Part model, mm, in its own coordinate system. A direction names the side the tool comes from. Coordinates: 2 decimals unless noted, no trailing zeros. Order: outer loops, then holes, each group sorted by start corner. A loop starts at its lowest first (then second) coordinate and runs counter-clockwise, first axis right, second up.
from build123d import *

# Parameters (mm, degrees)
SKETCH_1_R               = 19
EXTRUDE_1_DEPTH          = 69
CUT_EXTRUDE_1_DEPTH      = 75.047282192
CUT_EXTRUDE_1_DEPTH_BACK = 75.047282192
SKETCH_4_W               = 20
SKETCH_4_H               = 14
CUT_EXTRUDE_2_DEPTH      = 68.113709479
SKETCH_5_W               = 20
SKETCH_5_H               = 19.031424338
CUT_EXTRUDE_3_DEPTH      = 6
SKETCH_6_R               = 0.75
CUT_EXTRUDE_4_DEPTH      = 75.047282192
SKETCH_7_R               = 1.5
CUT_EXTRUDE_5_DEPTH      = 6.5


with BuildPart() as part:
    # 草图1 → 凸台-拉伸1 (new body)
    with BuildSketch(Plane(origin=(0, 0, 0), x_dir=(0, 0, -1), z_dir=(1, 0, 0))):
        Circle(SKETCH_1_R)
    extrude(amount=EXTRUDE_1_DEPTH)

    # 草图3 → 切除-拉伸1 (cut, two sides: drawn at the far end of the back side and taken through both)
    with BuildSketch(Plane.XY.offset(-CUT_EXTRUDE_1_DEPTH_BACK)):
        Polygon((69, 7.25), (61.5, 7.25), (61.5, -5.944695841), (47.305304159, -5.944695841), (40, -13.25), (0, -13.25), (0, 41.360608317), (69, 41.360608317), align=None)
    extrude(amount=CUT_EXTRUDE_1_DEPTH + CUT_EXTRUDE_1_DEPTH_BACK, mode=Mode.SUBTRACT)

    # 草图4 → 切除-拉伸2 (cut, through all)
    with BuildSketch(Plane.ZY.offset(-61.5)):
        with Locations((0, -6.25)):
            Rectangle(SKETCH_4_W, SKETCH_4_H)
    extrude(amount=CUT_EXTRUDE_2_DEPTH, mode=Mode.SUBTRACT)

    # 草图5 → 切除-拉伸3 (cut)
    with BuildSketch(Plane.ZY.offset(-61.5)):
        with Locations((0, -3.734287831)):
            Rectangle(SKETCH_5_W, SKETCH_5_H)
    extrude(amount=-CUT_EXTRUDE_3_DEPTH, mode=Mode.SUBTRACT)

    # 草图6 → 切除-拉伸4 (cut, through all)
    with BuildSketch(Plane(origin=(69, 0, 0), x_dir=(0, 0, -1), z_dir=(1, 0, 0))):
        with Locations((-13.2, 2.7)):
            Circle(SKETCH_6_R)
        with Locations((13.2, 2.7)):
            Circle(SKETCH_6_R)
    extrude(amount=-CUT_EXTRUDE_4_DEPTH, mode=Mode.SUBTRACT)

    # 草图7 → 切除-拉伸5 (cut)
    with BuildSketch(Plane(origin=(69, 0, 0), x_dir=(0, 0, -1), z_dir=(1, 0, 0))):
        with Locations((-13.2, 2.7)):
            Circle(SKETCH_7_R)
        with Locations((13.2, 2.7)):
            Circle(SKETCH_7_R)
    extrude(amount=-CUT_EXTRUDE_5_DEPTH, mode=Mode.SUBTRACT)


solid = part.part
Q1. Pin check, flat tips, straight feed: pin 1 Ø3 at (x, z) = (36, 7) entering from +Y; pin 2 Ø5 at (y, z) = (2.7, -13.2) entering from -X; pin 3 Ø4 at (x, z) = (53, 13) entering from +Y. Stop position of each tip, or through.
Results list:
pin 1: stops at y = -13.25
pin 2: stops at x = 61.5
pin 3: stops at y = -5.94
Q2. Cut at B-B on y = 0. Write the cut outline in (x, z), and give its area (3 significant figures).
Results list:
outline: (61.5, -19) - (69, -19) - (69, 19) - (61.5, 19) - (61.5, 10) - (67.5, 10) - (67.5, -10) - (61.5, -10) - close
area: 165 mm2
Q3. Mould opens along Y. For faces 5 (the face through (55, -5.945, 14)), 6 (the face through (65.8, 3.15, 11.77)), 7 (the face through (61.5, 7, 0)) say: pulls with the +Y half, pulls with the -Y half, needs draft (parallel to the pull), parting line crosses it, or undercut.
Results list:
face 5: pulls with the +Y half
face 6: undercut
face 7: needs draft
Q4. Cut at D-D on x = 12.5. Write the cut outline in (y, z), and give its area (3 significant figures).
Results list:
outline: (-13.25, -13.62) - (-13.25, 13.62) arc R19 ccw to start
area: 108 mm2
Q5. Cut at C-C on z = 0. Write the cut outline in (x, y), and give its area (3 significant figures).
Results list:
outline: (0, -19) - (69, -19) - (69, 7.25) - (61.5, 7.25) - (61.5, 5.78) - (67.5, 5.78) - (67.5, -13.25) - (0, -13.25) - close
area: 436 mm2
Q6. Wall check: line 1 along X through (y, z) = (3.25, 16); line 2 along Y through (x, z) = (61.75, -13.2); line 3 along X through (y, z) = (0.75, -4.5). Give the ranges that are in metal, low to high.
Results list:
line 1: x = 61.5 to 69
line 2: y = -13.67 to 1.95, 3.45 to 7.25
line 3: x = 67.5 to 69
Q7. Cut at A-A on x = 57.5. Write the cut outline in (y, z).
Results list:
outline: (-13.25, -10) - (-13.25, 10) - (-5.94, 10) - (-5.94, 18.05) arc R19 ccw to (-5.94, -18.05) - (-5.94, -10) - close
Q8. Which spindle directions (+Z, -Z, +X, -X, +Y, -Y) get a long thin tool onto all of the face, cutting with end or side? Do faces 1 (the face through (55, -5.945, -14)), 2 (the face through (62.5, 2, -14)), 3 (the face through (57, -8, -10)), 4 (the face through (62.01, 2.73, 13.95)). Say none if no direction does.
Results list:
face 1: +Z, -Z, -X, +Y
face 2: +X
face 3: -X
face 4: +X, -X
